Geometry check sheet. Reference: the model listing, model coordinates, mm. Coordinates: 2 decimals unless noted, no trailing zeros. Order: outer loops, then holes, each group sorted by start corner. A loop starts at its lowest first (then second) coordinate and runs counter-clockwise, first axis right, second up. Notation, with made-up numbers: (13, -19.75) - (30, -19.75) arc R21 cw to (30, 6.25) - close; hole circle Ø4 at (49.5, -24.75). An arc over 180 degrees is marked (long way). One line per item, written item: value. Start each with the question number.
```python
from build123d import *

# Parameters (mm, degrees)
F0_W     = 38.1
F0_H     = 571.5
F1_DEPTH = 19.05
F2_W     = 38.1
F2_H     = 38.1
F3_DEPTH = 9.525


with BuildPart() as f1:
    # F0 (on Right) → F1 (new body)
    with BuildSketch(Plane.YZ):
        with Locations((0, 207.162097)):
            Rectangle(F0_W, F0_H)
    extrude(amount=F1_DEPTH)

    # F2 (on face) → F3 (cut)
    with BuildSketch(Plane.YZ.offset(19.05)):
        with Locations((0, 473.862097)):
            Rectangle(F2_W, F2_H)
        with Locations((0, 181.762097)):
            Rectangle(F2_W, F2_H)
        with Locations((0, -59.537903)):
            Rectangle(F2_W, F2_H)
    extrude(amount=-F3_DEPTH, mode=Mode.SUBTRACT)


solid = f1.part
```
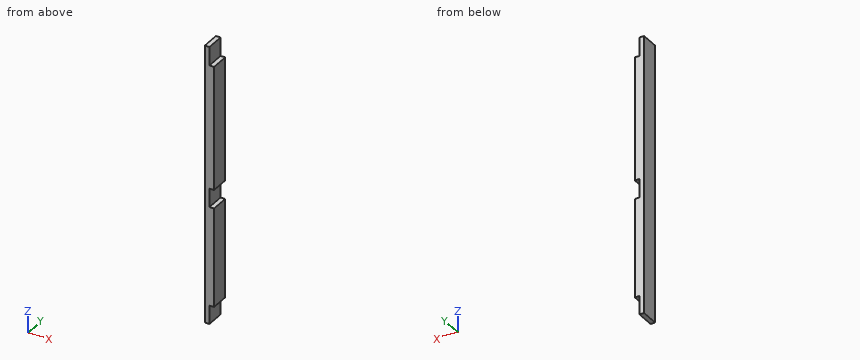
Q1. Gauge pin test, flat ends, axial feed: P1, Ø5, axis at x = 15.5, y = -0.5, coming from the -Z side; P2, Ø10.5, axis at x = 15, y = -3, coming from the +Z side; P3, Ø19, axis at y = -2, z = -56, coming from the +X side (3 decimals). Record the tip position at first contact, or that the pin passes through.
Q2. Cross-section at A-A, the plane x = 13.75. Enter the section's corners in (y, z).
Q3. Cross-section at B-B, the plane y = -9.5. Enter the section's corners in (x, z) (3 decimals), and give its area (3 significant figures).
Q4. Material ranges on probe 1 along Z at (x, y) = (15.25, 16), recorded low to high.
Check result:
1. P1: stops at z = -40.49
1. P2: stops at z = 454.81
1. P3: stops at x = 9.525
2. outline: (-19.05, -40.49) - (19.05, -40.49) - (19.05, 162.71) - (-19.05, 162.71) - close; (-19.05, 200.81) - (19.05, 200.81) - (19.05, 454.81) - (-19.05, 454.81) - close
3. outline: (0, -78.588) - (9.525, -78.588) - (9.525, -40.488) - (19.05, -40.488) - (19.05, 162.712) - (9.525, 162.712) - (9.525, 200.812) - (19.05, 200.812) - (19.05, 454.812) - (9.525, 454.812) - (9.525, 492.912) - (0, 492.912) - close
3. area: 9,800 mm2
4. probe 1: z = -40.49 to 162.71, 200.81 to 454.81
